```python
from build123d import *

# Parameters (mm, degrees)
F0_W      = 53.9978221059
F0_H      = 55.3920306265
F1_DEPTH  = 55.372
F2_W      = 55.3920306265
F2_H      = 55.372
F3_DEPTH  = 55.372
F4_W      = 55.3920306265
F4_H      = 55.372
F5_DEPTH  = 55.372
F6_W      = 53.9978221059
F6_H      = 55.3920306265
F7_DEPTH  = 55.372
F8_W      = 53.9978221059
F8_H      = 55.3920306265
F9_DEPTH  = 55.372
F10_W     = 55.3920306265
F10_H     = 67.3803910613
F11_DEPTH = 55.372


with BuildPart() as f1:
    # F0 (on Top) → F1 (new body)
    with BuildSketch(Plane.XY):
        with Locations((26.9989110529, -27.6960153133)):
            Rectangle(F0_W, F0_H)
    extrude(amount=F1_DEPTH)

    # F2 (on face) → F3 (join)
    with BuildSketch(Plane(origin=(0, 0, 0), x_dir=(0, -1, 0), z_dir=(-1, 0, 0))):
        with Locations((27.6960153133, 27.686)):
            Rectangle(F2_W, F2_H)
    extrude(amount=F3_DEPTH)

    # F4 (on face) → F5 (join)
    with BuildSketch(Plane(origin=(-55.372, 0, 0), x_dir=(0, -1, 0), z_dir=(-1, 0, 0))):
        with Locations((27.6960153133, 27.686)):
            Rectangle(F4_W, F4_H)
    extrude(amount=F5_DEPTH)

    # F6 (on face) → F7 (join)
    with BuildSketch(Plane(origin=(0, 0, 0), x_dir=(1, 0, 0), z_dir=(0, 0, -1))):
        with Locations((26.9989110529, 27.6960153133)):
            Rectangle(F6_W, F6_H)
    extrude(amount=F7_DEPTH)

    # F8 (on face) → F9 (join)
    with BuildSketch(Plane(origin=(0, 0, -55.372), x_dir=(1, 0, 0), z_dir=(0, 0, -1))):
        with Locations((26.9989110529, 27.6960153133)):
            Rectangle(F8_W, F8_H)
    extrude(amount=F9_DEPTH)

    # F10 (on face) → F11 (join)
    with BuildSketch(Plane(origin=(0, 0, 0), x_dir=(0, -1, 0), z_dir=(-1, 0, 0))):
        with Locations((27.6960153133, -33.6901955307)):
            Rectangle(F10_W, F10_H)
    extrude(amount=F11_DEPTH)


solid = f1.part
```
Geometry check sheet. Reference: the model listing, model coordinates, mm. A direction names the side the tool comes from. Round coordinates to 2 decimals unless told otherwise and drop trailing zeros. Loops run counter-clockwise (first coordinate to the right, second up) from the corner with the lowest first, then second, coordinate; pieces in that order, holes last. Notation, with made-up numbers: M 29,22.5 L 52,22.5 A8 cw 52,26.5 Z; hole C 10.25,79.25 d5. An arc over 180 degrees is marked long. Return JSON: item names as keys, results as strings. Group by question number.
(1) Section check B-B, the plane z = -82.5. Enter the section's corners in (x, y), and give its area (3 significant figures).
(2) Section check C-C, the plane x = -73.5. Enter the section's corners in (y, z).
(3) Section check A-A, the plane y = -6.5. Enter the section's corners in (x, z).
(4) Set-up check for faces 1 (the face through (-83, -27, 0)), 2 (the face through (53.998, -27, -27)): record each of +Z, -Z, +X, -X, +Y, -Y from which the full face is reachable in a straight line by a thin tool's end or side.
(5) Scan lines: line 1 along Z through (x, y) = (-16, -49.5); line 2 along X through (y, z) = (-52.5, -73.5); line 3 along X through (y, z) = (-23, -44). Record each from-to range of solid material in increasing order. Write a range as [from, to].
(6) Go/stop test with flat-tipped pins: pin 1 (13 mm diameter, centred on y = -26.5, z = -87.5, fed in from -X); pin 2 (4 mm diameter, centred on x = -30, y = -6.5, fed in from -Z); pin 3 (1 mm diameter, centred on x = -86, y = -38, fed in from -Z). Record where each tip stops, or that it passes through.
Data:
{
 "1": {"outline": "M 0,-55.39 L 54,-55.39 L 54,0 L 0,0 Z", "area": "2,990 mm²"},
 "2": {"outline": "M -55.39,0 L 0,0 L 0,55.37 L -55.39,55.37 Z"},
 "3": {"outline": "M -110.74,0 L -55.37,0 L -55.37,-67.38 L 0,-67.38 L 0,-110.74 L 54,-110.74 L 54,55.37 L -110.74,55.37 Z"},
 "4": {"face 1": "-Z, -X, +Y, -Y", "face 2": "+Z, -Z, +X, +Y, -Y"},
 "5": {"line 1": "[-67.38, 55.37]", "line 2": "[0, 54]", "line 3": "[-55.37, 54]"},
 "6": {"pin 1": "x = 0", "pin 2": "z = -67.38", "pin 3": "z = 0"}
}
